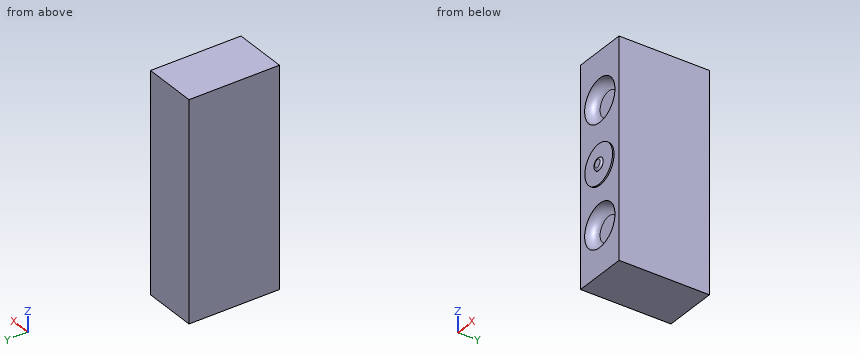
from build123d import *

# Parameters (mm, degrees)
F0_W     = 152.4
F0_H     = 254
F1_DEPTH = 609.6
F3_DEPTH = 25.4
F4_R     = 25.39999
F5_DEPTH = 4
F6_DEPTH = 8


# Not quite as in the source:
# - a fillet or chamfer that OpenCascade refuses, or shapes differently, is made with other operations: its cross-section is extruded or revolved along the edge and cut away or added
# - a fillet or chamfer is up to 0.001 mm smaller than in the source, because OpenCascade refuses the exact size


with BuildPart() as f1:
    # F0 (on Top) → F1 (new body)
    with BuildSketch(Plane.XY):
        with Locations((76.2, 127)):
            Rectangle(F0_W, F0_H)
    extrude(amount=F1_DEPTH)

    # F2 (on face) → F3 (cut)
    with BuildSketch(Plane.XZ):
        with BuildLine():
            Line((76.2, 414.5332613452), (76.2, 534.5332613452))
            ThreePointArc((76.2, 534.5332613452), (16.2, 474.5332613452), (76.2, 414.5332613452))
        make_face()
        with BuildLine():
            ThreePointArc((76.2, 414.5332613452), (118.6264068712, 432.106854474), (136.2, 474.5332613452))
            ThreePointArc((136.2, 474.5332613452), (118.6264068712, 516.9596682164), (76.2, 534.5332613452))
            Line((76.2, 534.5332613452), (76.2, 414.5332613452))
        make_face()
        with BuildLine():
            Line((76.2, 74.5332613452), (76.2, 194.5332613452))
            ThreePointArc((76.2, 194.5332613452), (16.2, 134.5332613452), (76.2, 74.5332613452))
        make_face()
        with BuildLine():
            ThreePointArc((136.2, 134.5332613452), (118.6264068712, 176.9596682164), (76.2, 194.5332613452))
            Line((76.2, 194.5332613452), (76.2, 74.5332613452))
            ThreePointArc((76.2, 74.5332613452), (118.6264068712, 92.106854474), (136.2, 134.5332613452))
        make_face()
    extrude(amount=-F3_DEPTH, mode=Mode.SUBTRACT)

    # F4 (radius 25.4 in the source; OpenCascade refuses exactly that, so slightly less here)
    f4_edges = [f1.edges().sort_by_distance(p)[0] for p in [
        (76.2, 25.4, 534.533261),
        (76.2, 25.4, 194.533261),
    ]]
    fillet(f4_edges, radius=F4_R)

    # F2 (on face) → F5 (join)
    with BuildSketch(Plane.XZ):
        with BuildLine():
            ThreePointArc((132.5678679347, 298.8973259926), (115.9720816592, 338.2688432126), (76.2, 353.8803137007))
            Line((76.2, 353.8803137007), (76.2, 316.3437851552))
            ThreePointArc((76.2, 316.3437851552), (89.4487835379, 311.7462109414), (95.0678679347, 298.8973259926))
            ThreePointArc((95.0678679347, 298.8973259926), (89.4487835379, 286.0484410437), (76.2, 281.45086683))
            Line((76.2, 281.45086683), (76.2, 243.9143382844))
            ThreePointArc((76.2, 243.9143382844), (115.9720816592, 259.5258087726), (132.5678679347, 298.8973259926))
        make_face()
        with BuildLine():
            Line((76.2, 316.3437851552), (76.2, 353.8803137007))
            ThreePointArc((76.2, 353.8803137007), (22.5678679347, 298.8973259926), (76.2, 243.9143382844))
            Line((76.2, 243.9143382844), (76.2, 281.45086683))
            ThreePointArc((76.2, 281.45086683), (60.0678679347, 298.8973259926), (76.2, 316.3437851552))
        make_face()
    extrude(amount=F5_DEPTH)

    # F2 (on face) → F6 (join)
    with BuildSketch(Plane.XZ):
        with BuildLine():
            ThreePointArc((95.0678679347, 298.8973259926), (89.4487835379, 311.7462109414), (76.2, 316.3437851552))
            Line((76.2, 316.3437851552), (76.2, 281.45086683))
            ThreePointArc((76.2, 281.45086683), (89.4487835379, 286.0484410437), (95.0678679347, 298.8973259926))
        make_face()
        with BuildLine():
            Line((76.2, 281.45086683), (76.2, 316.3437851552))
            ThreePointArc((76.2, 316.3437851552), (60.0678679347, 298.8973259926), (76.2, 281.45086683))
        make_face()
    extrude(amount=F6_DEPTH)

    # F7: fillet of radius 8 on 1 edges, made by hand

    # F7_s1 → F7_t2 (revolve, cut)
    with BuildSketch(Plane.XY.offset(298.8973259926)):
        with BuildLine():
            ThreePointArc((95.0678679347, -4), (92.1396647044, -6.9282032303), (88.1396647044, -8))
            Line((88.1396647044, -8), (95.0678679347, -8))
            Line((95.0678679347, -8), (95.0678679347, -4))
        make_face()
    revolve(axis=Axis((77.5678679347, -8, 298.8973259926), (0, -1, 0)), mode=Mode.SUBTRACT)


solid = f1.part
Design review of the part built by this model. Coordinates are the model's own, in mm. Give positions to 0.01 mm unless a question says otherwise; leave off trailing zeros. Write each loop counter-clockwise with the first axis right and the second up, starting at its lowest first coordinate (ties: lowest second). Pieces come first, ordered by that corner, then holes. Notation, with made-up numbers: M 86.25,-15.5 L 118.25,-15.5 A22 cw 118.25,-2.5 Z; hole C 51,-37 d8. An arc over 180 degrees is marked long. Answer as a JSON object with one key per item and string values. Group by question number.
1) We need section B-B (z = 562). Give the boundary of the cut face in (x, y), and give its area (3 significant figures).
2) Clearance check with flat-ended pins moving along their axes: pin 1 Ø1 at (x, z) = (43.5, 530.5) entering from -Y; pin 2 Ø6 at (x, z) = (91.5, 83) entering from -Y. State where each tip first meets the part, or that it passes through.
3) We need section A-A (x = 142.5). Give the boundary of the cut face in (y, z), and give its area (3 significant figures).
4) For line 1 along Y through (x, z) = (141.5, 405); line 2 along Y through (x, z) = (75, 325), list the stretches that pass through material, from the lowest coordinate up.
Answer key:
{
 "1": {"outline": "M 0,0 L 152.4,0 L 152.4,254 L 0,254 Z", "area": "38,700 mm²"},
 "2": {"pin 1": "stops at y = 0", "pin 2": "stops at y = 12.42"},
 "3": {"outline": "M 0,0 L 254,0 L 254,609.6 L 0,609.6 Z", "area": "155,000 mm²"},
 "4": {"line 1": "y = 0 to 254", "line 2": "y = -4 to 254"}
}
